Geometry: final body of the model. Coordinates: model frame, mm. Round coordinates to 2 decimals unless told otherwise and drop trailing zeros. Order: outer loops, then holes, each group sorted by start corner. A loop starts at its lowest first (then second) coordinate and runs counter-clockwise, first axis right, second up. Notation, with made-up numbers: M 24.5,3.25 L 79.5,3.25 A33 ccw 79.5,33.25 Z; hole C 23.25,61 d2. An arc over 180 degrees is marked long. Put each result on its own line as item: value. Start each with the question number.
1) Material intervals for probe 1 along Z at (x, y) = (18.5, -16.5); probe 2 along Z at (x, y) = (15.5, -20.5); probe 3 along X at (y, z) = (-28, 626.5) (3 decimals), sorted ascending. Write a range as [from, to].
2) Section B-B, the plane z = 64. Return loops of the section in (x, y).
3) Section A-A, the plane z = 145. Return loops of the section in (x, y) (3 decimals).
4) First-contact query: P1, Ø10, axis at x = 25.5, y = -24.5, coming from the -Z side; P2, Ø3, axis at x = 18.5, y = -14.5, coming from the +Z side. Flat tips, straight axial feed; report the tip coordinate or a pass-through.
from build123d import *

# Parameters (mm, degrees)
F1_DEPTH = 38.1
F2_SIZE2 = 76.2
F2_SIZE  = 6.35
F3_W     = 6.35
F3_H     = 38.1
F4_DEPTH = 38.101


with BuildPart() as f1:
    # F0 (on Front) → F1 (new body)
    with BuildSketch(Plane.XZ):
        Polygon((0, 660.4), (0, 0), (38.1, 0), (38.1, 660.4), (22.225, 660.4), (22.225, 622.3), (15.875, 622.3), (15.875, 660.4), align=None)
    extrude(amount=F1_DEPTH)

    # F2
    f2_edges = [f1.edges().sort_by_distance(p)[0] for p in [
        (19.05, -38.1, 0),
        (38.1, -19.05, 0),
        (19.05, 0, 0),
        (0, -19.05, 0),
    ]]
    f2_side = f1.faces().sort_by_distance((19.05, -19.05, 0))[0]
    chamfer(f2_edges, length=F2_SIZE, length2=F2_SIZE2, reference=f2_side)

    # F3 (on face) → F4 (cut, through all)
    with BuildSketch(Plane.YZ.offset(38.1)):
        with Locations((-19.05, 412.75)):
            Rectangle(F3_W, F3_H)
        with Locations((-19.05, 146.05)):
            Rectangle(F3_W, F3_H)
    extrude(amount=-F4_DEPTH, mode=Mode.SUBTRACT)


solid = f1.part
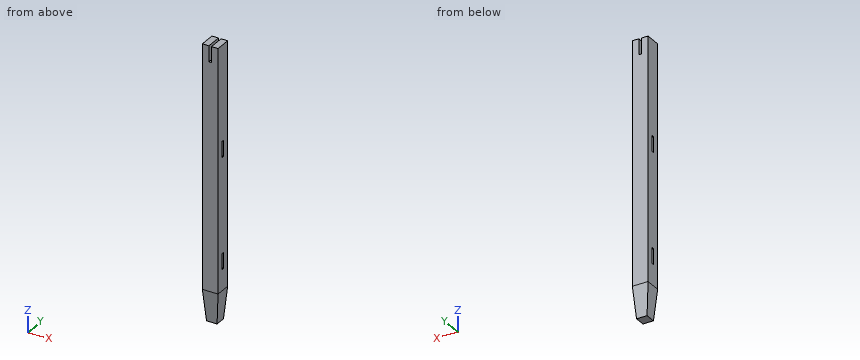
Result sheet:
1. probe 1: z = [0, 127], [165.1, 393.7], [431.8, 622.3]
1. probe 2: z = [0, 127], [165.1, 393.7], [431.8, 660.4]
1. probe 3: x = [0, 15.875], [22.225, 38.1]
2. outline: M 1.02,-37.08 L 37.08,-37.08 L 37.08,-1.02 L 1.02,-1.02 Z
3. outline: M 0,-38.1 L 38.1,-38.1 L 38.1,-22.225 L 0,-22.225 Z; M 0,-15.875 L 38.1,-15.875 L 38.1,0 L 0,0 Z
4. P1: stops at z = 0
4. P2: stops at z = 622.3
